```python
from build123d import *

# Parameters (mm, degrees)
ESQUISSE1_W             = 40
ESQUISSE1_H             = 5.1
BOSS_EXTRU_1_DEPTH      = 5
ENL_V_MAT_EXTRU_1_REACH = 7
BOSS_EXTRU_2_DEPTH      = 5


with BuildPart() as part:
    # Esquisse1 → Boss.-Extru.1 (new body)
    with BuildSketch(Plane.XY):
        Polygon((100, 330), (128.284271247, 301.715728753), (124.748737342, 298.180194847), (153.033008589, 269.895923599), (156.568542495, 273.431457505), (199.901875828, 230.098124172), (196.366341922, 226.562590266), (211.415404008, 211.51352818), (214.950937914, 215.049062086), (230, 200), (230, 160), (225, 160), (225, 120), (230, 120), (230, 80), (225, 80), (225, 40), (230, 40), (230, 0), (0, 0), (0, 50), (5, 50), (5, 100), (0, 100), (0, 150), (5, 150), (5, 200), (0, 200), (0, 250), (5, 250), (5, 300), (0, 300), (0, 350), (5, 350), (5, 400), (0, 400), (0, 450), (5, 450), (5, 500), (0, 500), (0, 550), (5, 550), (5, 600), (0, 600), (0, 650), (5, 650), (5, 700), (0, 700), (0, 750), (60, 750), (60, 745), (75, 745), (75, 750), (100, 750), (100, 700), (95, 700), (95, 650), (100, 650), (100, 600), (95, 600), (95, 550), (100, 550), (100, 500), (95, 500), (95, 450), (100, 450), (100, 400), (95, 400), (95, 350), (100, 350), align=None)
        with Locations((145, 232.55)):
            Rectangle(ESQUISSE1_W, ESQUISSE1_H, mode=Mode.SUBTRACT)
    extrude(amount=BOSS_EXTRU_1_DEPTH)

    # Esquisse3 → Enlèv. mat.-Extru.1 (cut, up to next)
    with BuildSketch(Plane.XY.offset(5), mode=Mode.PRIVATE) as enl_v_mat_extru_1_sk1:
        with BuildLine():
            Line((225, 156.507575951), (230, 156.507575951))
            Line((230, 156.507575951), (230, 200))
            Line((230, 200), (185.104076401, 244.895923599))
            Line((185.104076401, 244.895923599), (181.568542495, 241.360389693))
            Line((181.568542495, 241.360389693), (195.710678119, 227.218254069))
            ThreePointArc((195.710678119, 227.218254069), (217.387953251, 194.775919187), (225, 156.507575951))
        make_face()
    enl_v_mat_extru_1_tool1 = extrude(enl_v_mat_extru_1_sk1.sketch, amount=-ENL_V_MAT_EXTRU_1_REACH, mode=Mode.PRIVATE) & part.part
    add(enl_v_mat_extru_1_tool1.solids().sort_by_distance((215.711514, 201.173028, 5))[0], mode=Mode.SUBTRACT)

    # Esquisse4 → Boss.-Extru.2 (add)
    with BuildSketch(Plane.XY.offset(5)):
        with BuildLine():
            Line((100, 350), (100, 330))
            Line((100, 330), (114.142135624, 315.857864376))
            ThreePointArc((114.142135624, 315.857864376), (103.6754213, 331.52240935), (100, 350))
        make_face()
    extrude(amount=-BOSS_EXTRU_2_DEPTH)


solid = part.part
```
Part model, mm, in its own coordinate system. A direction names the side the tool comes from. Round coordinates to 2 decimals unless told otherwise and drop trailing zeros. Write each loop counter-clockwise with the first axis right and the second up, starting at its lowest first coordinate (ties: lowest second). Pieces come first, ordered by that corner, then holes. Notation, with made-up numbers: (4, 50.25) -> (63, 50.25) arc R29 cw to (63, 73.25) -> close; hole circle Ø1 at (-34.5, -6.5). An arc over 180 degrees is marked (long way). Return JSON: item names as keys, results as strings. Group by question number.
Q1. Saw through at A-A on y = 531. Write the cut outline in (x, z), plus the area to 3 significant figures.
Q2. Probe L1, parallel to Y at x = 149.5, z = 4.65; L2, parallel to X at y = 689.5, z = 2.8; L3, parallel to X at y = 245, z = 2.3. List the from-to ranges inside material, lowest first. Write a range as [from, to].
Q3. Pin check, flat tips, straight feed: pin 1 (1.5 mm diameter, centred on y = 584.5, z = 2, fed in from +X); pin 2 (3 mm diameter, centred on y = 339, z = 4, fed in from +X); pin 3 (3 mm diameter, centred on y = 263.5, z = 3.5, fed in from -X). Stop position of each tip, or through.
Q4. Which spindle directions (+Z, -Z, +X, -X, +Y, -Y) get a long thin tool onto all of the face, cutting with end or side? Do faces 1 (the flat face through (188.54, 234.39, 2.54)), 2 (the cylindrical face through (217.176, 195.283, 2.535)). Say none if no direction does.
Q5. Saw through at B-B on x = 213. Write the cut outline in (y, z), plus the area to 3 significant figures.
Answer:
{
 "1": {"outline": "(0, 0) -> (100, 0) -> (100, 5) -> (0, 5) -> close", "area": "500 mm2"},
 "2": {"L1": "[0, 230], [235.1, 273.43]", "L2": "[5, 95]", "L3": "[0, 185]"},
 "3": {"pin 1": "x = 95", "pin 2": "x = 101.65", "pin 3": "x = 5"},
 "4": {"face 1": "+Z, -Z, +X", "face 2": "+Z, -Z, +X, +Y"},
 "5": {"outline": "(0, 0) -> (204, 0) -> (204, 5) -> (0, 5) -> close", "area": "1,020 mm2"}
}
